Part model, mm, in its own coordinate system. Give positions to 0.01 mm unless a question says otherwise; leave off trailing zeros. Write each loop counter-clockwise with the first axis right and the second up, starting at its lowest first coordinate (ties: lowest second). Pieces come first, ordered by that corner, then holes. Notation, with made-up numbers: M 78,80.5 L 89,80.5 A29 ccw 89,115.5 Z; hole C 86,-38 d8. An arc over 180 degrees is marked long. Use a Markdown table: item, result.
Solid Edge part; units mm, degrees
sketch "Sketch1" plane through (0, 0, 0) normal (0, 0, 1) x (1, 0, 0)
  line L0 (-183.0017, -120) -> (-227.4217, -120)
  line L1 (-289.5811, -57.8353) -> (-227.4217, -120)
  line L2 (-289.5811, -57.8353) -> (-351.7458, 4.3295)
  line L3 (-351.7458, 129.7437) -> (-351.7458, 4.3295)
  line L4 (-351.7458, 129.7437) -> (-351.7458, 255.1579)
  line L5 (-289.4346, 317.4691) -> (-351.7458, 255.1579)
  line L6 (-289.4346, 317.4691) -> (-227.7006, 379.2031)
  line L7 (0, 379.2031) -> (-227.7006, 379.2031)
  line L8 (0, 379.2031) -> (0, 0)
  line L9 (0, 0) -> (-183.0017, 0)
  line L10 (-183.0017, 0) -> (-183.0017, -120)
  dimension "D1" = 183.0017
  dimension "D2" = 183.0017
  dimension "D3" = 289.4346
  dimension "D4" = 289.4346
  dimension "D5" = 351.7458
  dimension "D6" = 351.7458
  dimension "D7" = 289.5811
  dimension "D8" = 289.5811
extrude "Protrusion1" add sketch "Sketch1" along normal blind 5
mirror "Mirror1" about plane through (0, 0, 0) normal (1, 0, 0) of "Protrusion1"
sketch "Sketch2" plane through (0, 149.6016, 5) normal (0, 0, 1) x (1, 0, 0)
  circle A0 centre (150, 209.6016) radius 4
  circle A1 centre (-150, 209.6016) radius 4
extrude "Cutout1" cut sketch "Sketch2" against normal through all
sketch "Sketch3" plane through (0, 149.6016, 5) normal (0, 0, 1) x (1, 0, 0)
  circle A0 centre (-331.7458, 60.1421) radius 4
  circle A1 centre (-331.7458, -99.8579) radius 4
  dimension "D1" = 331.7458
extrude "Cutout2" cut sketch "Sketch3" against normal through all
mirror "Mirror2" about plane through (0, 0, 0) normal (1, 0, 0) of "Cutout2"
sketch "Sketch4" plane through (0, 149.6016, 0) normal (0, 0, -1) x (-1, 0, 0)
  line L0 (-351.7458, -111.1142) -> (-193.1203, -269.6016)
  line L1 (-193.1203, -269.6016) -> (-227.4217, -269.6016)
  arc A0 (-351.7458, -145.2721) -> (-227.4217, -269.6016) centre (-220.2414, -138.0974) ccw
  line L2 (-351.7458, -111.1142) -> (-351.7458, -145.2721)
extrude "Protrusion2" add sketch "Sketch4" against normal up to vertex (5 mm away)
sketch "Sketch5" plane through (0, 149.6016, 0) normal (0, 0, -1) x (-1, 0, 0)
  line L0 (-227.7006, 229.6016) -> (-351.7458, 105.5563)
  arc A0 (-351.7458, 105.5563) -> (-227.7006, 229.6016) centre (-220.2564, 98.1121) cw
extrude "Protrusion3" add sketch "Sketch5" against normal up to vertex (5 mm away)
mirror "Mirror3" about plane through (0, 0, 0) normal (1, 0, 0) of "Protrusion3", "Protrusion2"
properties material "ABS-Plastik, mittelfest"
1. Drop flat-ended pins along their axis: P1, Ø2.5, axis at x = -25, z = 3.5, coming from the -Y side; P2, Ø1.5, axis at y = -60.5, z = 1.5, coming from the +X side; P3, Ø1.5, axis at x = -82, y = -0.5, coming from the -Z side; P4, Ø2.5, axis at y = -42, z = 2.5, coming from the -X side. Give the stop position or say it passes through.
Findings below:
| item | result |
|---|---|
| P1 | y = 0 |
| P2 | x = 331 |
| P3 | z = 0 |
| P4 | x = -341.13 |
2. Cut at A-A, the plane z = 2.8. Give the cut face in (x, y).
Findings below:
| item | result |
|---|---|
| outline | M -351.75,4.33 A131.7 ccw -227.42,-120 L -183,-120 L -183,0 L 183,0 L 183,-120 L 227.42,-120 A131.7 ccw 351.75,4.33 L 351.75,255.16 A131.7 ccw 227.7,379.2 L -227.7,379.2 A131.7 ccw -351.75,255.16 Z; hole C -331.75,49.74 d8; hole C -331.75,209.74 d8; hole C -150,359.2 d8; hole C 150,359.2 d8; hole C 331.75,49.74 d8; hole C 331.75,209.74 d8 |
3. Drill centre lines: L1, parallel to Y at x = -150, z = 3.4; L2, parallel to Y at x = -19.5, z = 0.9; L3, parallel to X at y = 212.5, z = 0.7. Where is each one in solid material? Low to high.
Findings below:
| item | result |
|---|---|
| L1 | 0 to 355.2, 363.2 to 379.2 |
| L2 | 0 to 379.2 |
| L3 | -351.75 to -334.64, -328.85 to 328.85, 334.64 to 351.75 |
4. Cut at B-B, the plane y = 311.5. Give the cut face in (x, z), then the cut area to 3 significant figures.
Findings below:
| item | result |
|---|---|
| outline | M -335.48,0 L 335.48,0 L 335.48,5 L -335.48,5 Z |
| area | 3,350 mm2 |
